from build123d import *

# Parameters (mm, degrees)
F0_R     = 38.1
F1_DEPTH = 12.7
F2_W     = 42.448588
F2_H     = 91.320313
F3_DEPTH = 12.7
F4_R     = 4
F5_DEPTH = 38.101


with BuildPart() as f1:
    # F0 (on Top) → F1 (new body)
    with BuildSketch(Plane.XY):
        Circle(F0_R)
    extrude(amount=F1_DEPTH)

    # F2 (on face) → F3 (cut, through all)
    with BuildSketch(Plane.XY.offset(12.7)):
        with Locations((-21.224294, 1.396335)):
            Rectangle(F2_W, F2_H)
    extrude(amount=-F3_DEPTH, mode=Mode.SUBTRACT)

    # F4 (on face) → F5 (cut, through all)
    with BuildSketch(Plane(origin=(0, 0, 0), x_dir=(0, -1, 0), z_dir=(-1, 0, 0))):
        with Locations((-31.75, 6.35)):
            Circle(F4_R)
        with Locations((-19.05, 6.35)):
            Circle(F4_R)
        with Locations((-6.35, 6.35)):
            Circle(F4_R)
        with Locations((6.35, 6.35)):
            Circle(F4_R)
        with Locations((19.05, 6.35)):
            Circle(F4_R)
        with Locations((31.75, 6.35)):
            Circle(F4_R)
    extrude(amount=-F5_DEPTH, mode=Mode.SUBTRACT)


solid = f1.part
Build history of the part. All positions in model axes, mm. Coordinates: 2 decimals unless noted, no trailing zeros. Order: outer loops, then holes, each group sorted by start corner. A loop starts at its lowest first (then second) coordinate and runs counter-clockwise, first axis right, second up. Notation, with made-up numbers: (-20.5, 63) - (0.5, 63) arc R9 ccw to (0.5, 80) - close; hole circle Ø4 at (81, -9.5). An arc over 180 degrees is marked (long way). Put each result on its own line as item: value.
1. Saw through at D-D (x = 14.5). Write the cut outline in (y, z), and give its area (3 significant figures).
Answer sheet:
outline: (-35.23, 0) - (35.23, 0) - (35.23, 4.38) arc R4 cw (long way) to (35.23, 8.32) - (35.23, 12.7) - (-35.23, 12.7) - (-35.23, 8.32) arc R4 cw (long way) to (-35.23, 4.38) - close; hole circle Ø8 at (-19.05, 6.35); hole circle Ø8 at (-6.35, 6.35); hole circle Ø8 at (6.35, 6.35); hole circle Ø8 at (19.05, 6.35)
area: 596 mm^2
2. Saw through at B-B (x = 34). Write the cut outline in (y, z).
Answer sheet:
outline: (-17.19, 0) - (17.19, 0) - (17.19, 2.81) arc R4 cw to (17.19, 9.89) - (17.19, 12.7) - (-17.19, 12.7) - (-17.19, 9.89) arc R4 cw to (-17.19, 2.81) - close; hole circle Ø8 at (-6.35, 6.35); hole circle Ø8 at (6.35, 6.35)
3. Drop flat-ended pins along their axis: P1, Ø2, axis at x = 24.5, z = 3, coming from the -Y side; P2, Ø5, axis at y = 31.75, z = 6.35, coming from the +X side; P3, Ø1, axis at x = 15, z = 10.5, coming from the +Y side; P4, Ø5, axis at x = 24.5, z = 11.5, coming from the +Y side. Give the stop position or say it passes through.
Answer sheet:
P1: stops at y = -29.97
P2: passes through
P3: stops at y = 35.23
P4: stops at y = 31.11
4. Pull direction Z, two halves, no side cores. Call faces 1 (the face through (18.75, -8.5, 9.723)), 2 (the face through (0, -1, 6)), 3 (the face through (15, 1, 12.7)), 4 (the face through (17.256, 15.235, 7.551)): pulls with the +Z half, pulls with the -Z half, needs draft (parallel to the pull), parting line crosses it, or undercut.
Answer sheet:
face 1: undercut
face 2: needs draft
face 3: pulls with the +Z half
face 4: undercut
5. Probe line 1 along Y through (x, z) = (20, 6.35); line 2 along Z through (x, y) = (28, 19); line 3 along Z through (x, y) = (9, -17.5). List the from-to ranges inside material, lowest first. Write a range as [from, to].
Answer sheet:
line 1: y = [-27.75, -23.05], [-15.05, -10.35], [-2.35, 2.35], [10.35, 15.05], [23.05, 27.75]
line 2: z = [0, 2.35], [10.35, 12.7]
line 3: z = [0, 2.66], [10.04, 12.7]
6. Saw through at C-C (y = -19.05). Write the cut outline in (x, z).
Answer sheet:
outline: (0, 0) - (33, 0) - (33, 2.35) - (0, 2.35) - close; (0, 10.35) - (33, 10.35) - (33, 12.7) - (0, 12.7) - close
7. Saw through at A-A (y = 31.75). Write the cut outline in (x, z), and give its area (3 significant figures).
Answer sheet:
outline: (0, 0) - (21.06, 0) - (21.06, 2.35) - (0, 2.35) - close; (0, 10.35) - (21.06, 10.35) - (21.06, 12.7) - (0, 12.7) - close
area: 99.0 mm^2
